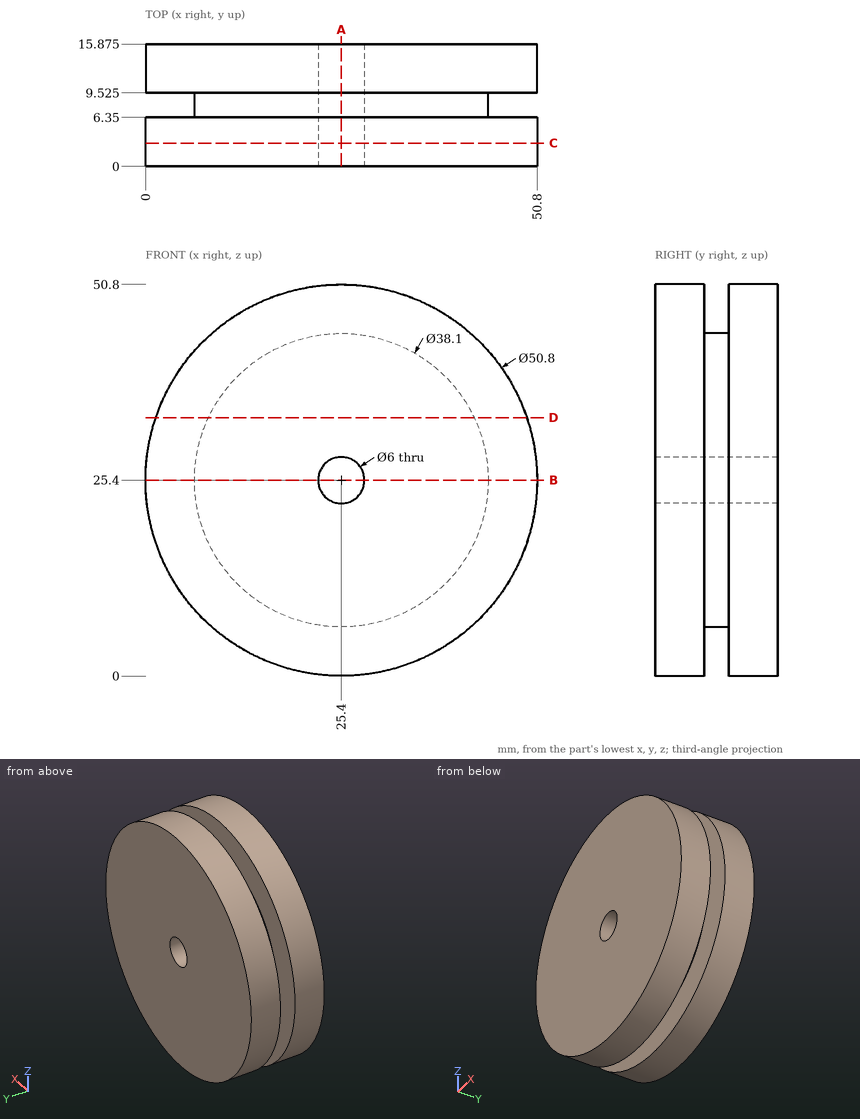
The figure shows three views and two pictorial views of one solid part (mm, origin at its lowest corner). Answer the questions. Give positions to 0.01 mm unless a question says otherwise; leave off trailing zeros. Write each loop counter-clockwise with the first axis right and the second up, starting at its lowest first coordinate (ties: lowest second). Pieces come first, ordered by that corner, then holes. Notation, with made-up numbers: M 54,-39 L 97,-39 A15 cw 97,-15 Z; hole C 11.5,17.25 d7. An arc over 180 degrees is marked long. One line per item, written item: value. Start each with the question number.
(1) Find section D-D (z = 33.5). Determine the outline of the cut face in (x, y) (3 decimals).
(2) Flat-ended cylindrical pins translate along their axes: pin 1 Ø1 at (x, y) = (6, 13) entering from -Z; pin 2 Ø3 at (x, y) = (33.5, 6) entering from -Z; pin 3 Ø4 at (x, y) = (9, 5) entering from -Z. Find the tip coordinate at first contact, or state that the pin passes through.
(3) Find section A-A (x = 25.4). Determine the outline of the cut face in (y, z) (3 decimals).
(4) Find the intervals of material crossed by line 1 (Y direction, x = 46, z = 22) (3 decimals); line 2 (Z direction, x = 25.4, y = 11); line 3 (X direction, y = 6.5, z = 25.4), in increasing order.
(5) Find section B-B (z = 25.4). Determine the outline of the cut face in (x, y) (3 decimals), plus the area to 3 significant figures.
(6) Find section C-C (y = 3). Determine the outline of the cut face in (x, z), plus the area to 3 significant figures.
Results below:
1. outline: M 1.326,0 L 49.474,0 L 49.474,6.35 L 42.642,6.35 L 42.642,9.525 L 49.474,9.525 L 49.474,15.875 L 1.326,15.875 L 1.326,9.525 L 8.158,9.525 L 8.158,6.35 L 1.326,6.35 Z
2. pin 1: stops at z = 8.43
2. pin 2: stops at z = 0.87
2. pin 3: stops at z = 4.48
3. outline: M 0,0 L 6.35,0 L 6.35,6.35 L 9.525,6.35 L 9.525,0 L 15.875,0 L 15.875,22.4 L 0,22.4 Z; M 0,28.4 L 15.875,28.4 L 15.875,50.8 L 9.525,50.8 L 9.525,44.45 L 6.35,44.45 L 6.35,50.8 L 0,50.8 Z
4. line 1: y = 0 to 6.35, 9.525 to 15.875
4. line 2: z = 0 to 22.4, 28.4 to 50.8
4. line 3: x = 6.35 to 22.4, 28.4 to 44.45
5. outline: M 0,0 L 22.4,0 L 22.4,15.875 L 0,15.875 L 0,9.525 L 6.35,9.525 L 6.35,6.35 L 0,6.35 Z; M 28.4,0 L 50.8,0 L 50.8,6.35 L 44.45,6.35 L 44.45,9.525 L 50.8,9.525 L 50.8,15.875 L 28.4,15.875 Z
5. area: 671 mm^2
6. outline: C 25.4,25.4 d50.8; hole C 25.4,25.4 d6
6. area: 2,000 mm^2
